Geometry: final body of the model. Coordinates: model frame, mm. Round coordinates to 2 decimals unless told otherwise and drop trailing zeros. Order: outer loops, then holes, each group sorted by start corner. A loop starts at its lowest first (then second) coordinate and runs counter-clockwise, first axis right, second up. Notation, with made-up numbers: M -25.5,60.25 L -19.5,60.25 A29 cw -19.5,91.25 Z; hole C -21.5,-10 d9. An arc over 180 degrees is marked long. Return JSON: item names as keys, results as strings. Group by question number.
Q1. Cut plane C-C on y = 25. Output: boundary loops of the cut face in (x, z), and give its area (3 significant figures).
Q2. Cut plane D-D on z = 1.75. Output: boundary loops of the cut face in (x, y), and give its area (3 significant figures).
Q3. Cut plane B-B on y = 60. Output: boundary loops of the cut face in (x, z).
Q4. Ray query, probe 1 along Y at (x, z) = (164, 1); probe 2 along X at (y, z) = (24.5, 2.85); probe 3 along X at (y, z) = (24, 1.5). Return the intervals inside material, ascending.
Q5. Contact query for flat-ended pins moving along their axis: pin 1 (1 mm diameter, centred on y = 45.5, z = 2, fed in from -X); pin 2 (1 mm diameter, centred on y = 57.5, z = 1.5, fed in from -X). Output: stop coordinate, or through.
Q6. Mould query, pull axis X, two halves, no side actions, for faces 1 (the face through (162, 60, 1)), 2 (the face through (161.669, 24.474, 1.479)), 3 (the face through (160.807, 41.429, 1.479)), 4 (the face through (157.271, 22.076, 1.479)). Classes: released by +X, released by -X, zero draft, split by the parting line, or undercut.
Q7. Cut plane A-A on x = 155.5. Output: boundary loops of the cut face in (y, z).
Autodesk Inventor part; units mm, degrees
ref_plane "YZ Plane" through (0, 0, 0) normal (1, 0, 0) x (0, 1, 0)
ref_plane "XZ Plane" through (0, 0, 0) normal (0, 1, 0) x (-1, 0, 0)
ref_plane "XY Plane" through (0, 0, 0) normal (0, 0, 1) x (1, 0, 0)
sketch "スケッチ1" plane through (0, 0, 0) normal (0, 0, 1) x (1, 0, 0)
  line L0 (160, 60) -> (160, 25) construction
  line L1 (160, 25) -> (154.8697, 39.0954) construction
  line L2 (154.8697, 39.0954) -> (174.0726, 33.5055) construction
  line L3 (174.0726, 33.5055) -> (160, 60) construction
  circle A0 centre (154.8697, 39.0954) radius 3 construction
  circle A1 centre (160, 60) radius 4 construction
  circle A2 centre (160, 60) radius 8
  line L4 (161.8764, 56.4674) -> (158.1236, 63.5326) construction
  circle A3 centre (164, 60) radius 4 construction
  circle A4 centre (156, 60) radius 4 construction
  circle A5 centre (164, 60) radius 3
  circle A6 centre (156, 60) radius 3
  line L5 (164, 60) -> (156, 60) construction
  circle A7 centre (160, 25) radius 4
  circle A8 centre (160, 25) radius 1.75
  arc A9 (162.5102, 21.8857) -> (165.9333, 65.3662) centre (143.6835, 45.2429) ccw
  arc A10 (156.8162, 27.4214) -> (154.542, 54.151) centre (140.8971, 39.5286) ccw
  circle A11 centre (156, 60) radius 2
  circle A12 centre (164, 60) radius 2
  point P0 (0, 0)
  point P1 (136.5819, 50.9264)
  point P2 (160, 60)
  dimension "d0" = 15
  dimension "d1" = 20
  dimension "d2" = 30
  dimension "d3" = 35
  dimension "d4" = 6
  dimension "d5" = 340
  dimension "d6" = 16
  dimension "d7" = 8
  dimension "d8" = 6
  dimension "d9" = 6
  dimension "d10" = 8
  dimension "d11" = 3.5
  dimension "d12" = 20
  dimension "d15" = 4
  dimension "d16" = 4
  dimension "d17" = 30
extrude "押し出し1" add sketch "スケッチ1" along normal blind 3 contours A2 | A2 A9 A7 A10 | A7 | A5 | A6
properties part number "原動節外側" material "アルミニウム 2014-T4"
Result sheet:
{
 "1": {"outline": "M 156,0 L 158.25,0 L 158.25,3 L 156,3 Z; M 161.75,0 L 165.82,0 L 165.82,3 L 161.75,3 Z", "area": "19.0 mm²"},
 "2": {"outline": "M 154.54,54.15 A20 cw 156.82,27.42 A4 ccw 162.51,21.89 A30 ccw 165.93,65.37 A8 ccw long Z; hole C 156,60 d4; hole C 160,25 d3.5; hole C 164,60 d4", "area": "579 mm²"},
 "3": {"outline": "M 152,0 L 154,0 L 154,3 L 152,3 Z; M 158,0 L 162,0 L 162,3 L 158,3 Z; M 166,0 L 169.8,0 L 169.8,3 L 166,3 Z"},
 "4": {"probe 1": "y = 23.17 to 58, 62 to 66.93", "probe 2": "x = 156.03 to 158.32, 161.68 to 165.36", "probe 3": "x = 156.13 to 158.56, 161.44 to 164.87"},
 "5": {"pin 1": "stops at x = 159.82", "pin 2": "stops at x = 152.25"},
 "6": {"face 1": "undercut", "face 2": "undercut", "face 3": "released by -X", "face 4": "split by the parting line"},
 "7": {"outline": "M 53.19,0 L 58.06,0 L 58.06,3 L 53.19,3 Z; M 61.94,0 L 66.61,0 L 66.61,3 L 61.94,3 Z"}
}
